```python
from build123d import *

# Parameters (mm, degrees)
BOSS_EXTRUDE1_DEPTH = 34
SWEEP2_PROFILE_R    = 1
LPATTERN1_COUNT     = 2
LPATTERN1_PITCH     = 4


with BuildPart() as part:
    # Sketch1 → Boss-Extrude1 (new body)
    with BuildSketch(Plane(origin=(0, 0, 0), x_dir=(1, 0, 0), z_dir=(0, 1, 0))):
        with BuildLine():
            Line((0, 0), (63, 0))
            Line((63, 0), (63, 24))
            Line((63, 24), (0, 24))
            ThreePointArc((0, 24), (-12, 12), (0, 0))
        make_face()
    extrude(amount=BOSS_EXTRUDE1_DEPTH)

    # Sweep2: sweep along a path in Sketch21
    with BuildLine(Plane(origin=(0, 0, -14), x_dir=(-1, 0, 0), z_dir=(0, 0, -1))) as sweep2_path:
        ThreePointArc((6, 34), (8.626551961, 38.989949378), (14.22684679, 39.649546094))
    # Sweep2 profile (on start of the path) → Sweep2 (sweep)
    with BuildSketch(Plane(origin=(-6, 34, -14), x_dir=(1, 0, 0), z_dir=(0, 1, 0))):
        Circle(SWEEP2_PROFILE_R)
    sweep2 = sweep(path=sweep2_path.line)

    # LPattern1: Sweep2 ×2
    with Locations(*[(0, 0, i * LPATTERN1_PITCH) for i in range(1, LPATTERN1_COUNT)]):
        add(sweep2)


solid = part.part
```
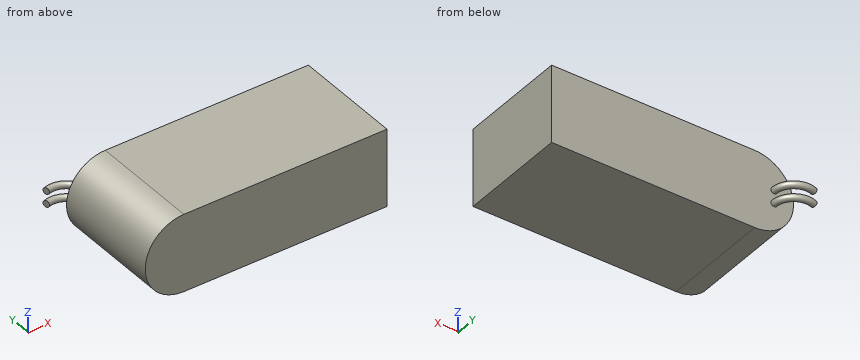
Verification items for the finished model (mm, model axes). Coordinates: 2 decimals unless noted, no trailing zeros. Loops run counter-clockwise (first coordinate to the right, second up) from the corner with the lowest first, then second, coordinate; pieces in that order, holes last. Notation, with made-up numbers: (87.25, -8.5) -> (142.25, -8.5) arc R15 ccw to (142.25, 6.5) -> close; hole circle Ø1 at (78.25, -22.5). An arc over 180 degrees is marked (long way). Answer in a Markdown table with one row per item.
1) Depth check by flat-ended pin: P1, Ø1.5, axis at x = 34, z = -5, coming from the +Y side; P2, Ø1.5, axis at y = 10, z = -9.5, coming from the -X side. Enter the tip coordinate at first touch or a pass-through.
The answers:
| item | result |
|---|---|
| P1 | stops at y = 34 |
| P2 | stops at x = -11.87 |
2) Section check A-A (y = 27.5). Record the cut outline in (x, z).
The answers:
| item | result |
|---|---|
| outline | (0, -24) -> (63, -24) -> (63, 0) -> (0, 0) arc R12 ccw to start |
3) Scan lines: line 1 along Y through (x, z) = (41, -5.5); line 2 along X through (y, z) = (11, -12.5); line 3 along X through (y, z) = (22, -8.25). Record each from-to range of solid material in increasing order. Write a range as from..to.
The answers:
| item | result |
|---|---|
| line 1 | y = 0..34 |
| line 2 | x = -11.99..63 |
| line 3 | x = -11.4..63 |
4) Section check B-B (z = -12). Record the cut outline in (x, y).
The answers:
| item | result |
|---|---|
| outline | (-12, 0) -> (63, 0) -> (63, 34) -> (-12, 34) -> close |
